Job drawing, mm, ordinate dimensions from the low corner. One solid piece. A direction names the side the tool comes from. Give positions to 0.01 mm unless a question says otherwise; leave off trailing zeros. Write each loop counter-clockwise with the first axis right and the second up, starting at its lowest first coordinate (ties: lowest second). Pieces come first, ordered by that corner, then holes. Notation, with made-up numbers: M -26.75,42 L -7.75,42 A18 cw -7.75,75 Z; hole C 31.5,78 d2. An arc over 180 degrees is marked long. Use a Markdown table: item, result.
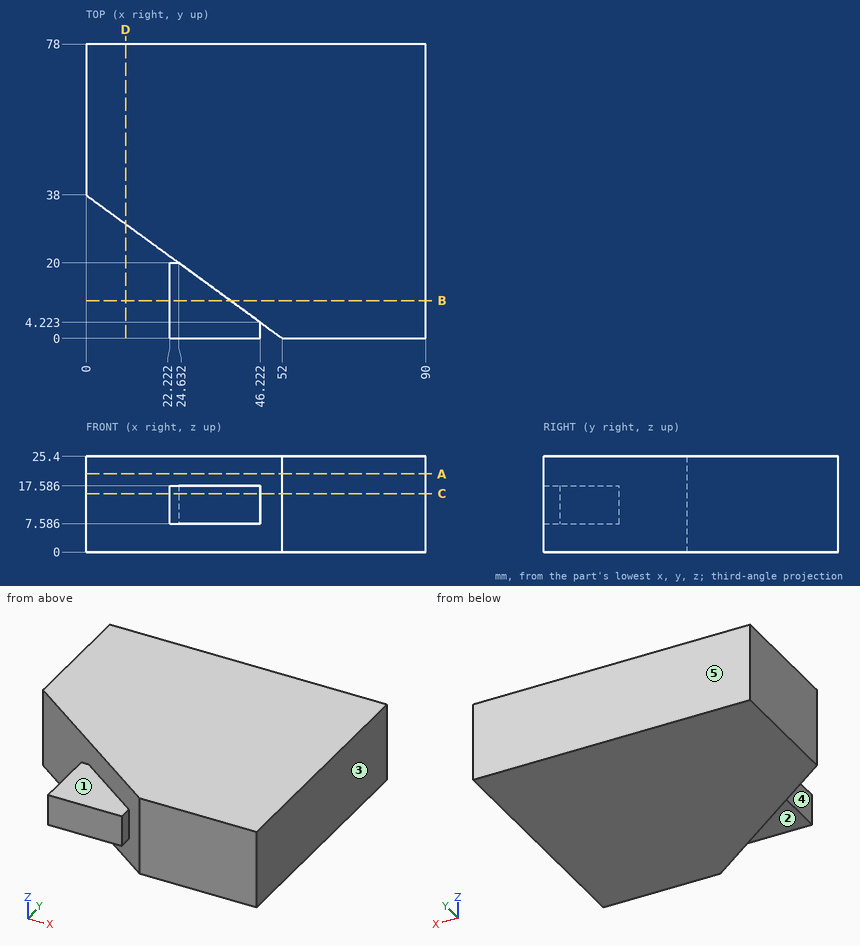
1. Cut at A-A, the plane z = 20.75. Give the cut face in (x, y).
Findings below:
| item | result |
|---|---|
| outline | M 0,38 L 52,0 L 90,0 L 90,78 L 0,78 Z |
2. Drop flat-ended pins along their axis: P1, Ø16, axis at x = 30.5, y = 6.5, coming from the -Z side; P2, Ø6, axis at x = 13, z = 3.5, coming from the -Y side; P3, Ø5, axis at y = 18.5, z = 18.5, coming from the -X side. Give the stop position or say it passes through.
Findings below:
| item | result |
|---|---|
| P1 | z = 0 |
| P2 | y = 26.31 |
| P3 | x = 22.22 |
3. Cut at C-C, the plane z = 15.5. Give the cut face in (x, y), then the cut area to 3 significant figures.
Findings below:
| item | result |
|---|---|
| outline | M 0,38 L 24.63,20 L 22.22,20 L 22.22,0 L 46.22,0 L 46.22,4.22 L 52,0 L 90,0 L 90,78 L 0,78 Z |
| area | 6,340 mm2 |
4. Cut at B-B, the plane y = 10. Give the cut face in (x, z) (1 decimal).
Findings below:
| item | result |
|---|---|
| outline | M 22.2,7.6 L 38.3,7.6 L 38.3,0 L 90,0 L 90,25.4 L 38.3,25.4 L 38.3,17.6 L 22.2,17.6 Z |
5. Tool access for the marked faces 1, 2, 3, 4 and 5: list every direction of +Z, -Z, +X, -X, +Y, -Y with a clear straight run to the whole face (end or side of a thin tool).
Findings below:
| item | result |
|---|---|
| face 1 | +Z, -X, -Y |
| face 2 | -Z, -X, -Y |
| face 3 | +Z, -Z, +X, +Y, -Y |
| face 4 | +Z, -Z, -X, -Y |
| face 5 | +Z, -Z, +X, -X, +Y |
6. Drill centre lines: L1, parallel to X at y = 13, z = 15; L2, parallel to X at y = 14, z = 3.5 (1 decimal); L3, parallel to Y at x = 30, z = 2.5 (1 decimal). Where is each one in solid material? Low to high.
Findings below:
| item | result |
|---|---|
| L1 | 22.22 to 90 |
| L2 | 32.8 to 90 |
| L3 | 16.1 to 78 |
7. Cut at D-D, the plane x = 10.5. Give the cut face in (y, z).
Findings below:
| item | result |
|---|---|
| outline | M 30.33,0 L 78,0 L 78,25.4 L 30.33,25.4 Z |
